Autodesk Fusion 360 part; units mm, degrees
sketch "スケッチ2" plane through (0, 0, 0) normal (0, 0, 1) x (1, 0, 0)
  line L0 (27.5, 37.5) -> (27.5, -37.5)
  line L1 (-27.5, -37.5) -> (-27.5, 37.5)
  arc A0 (27.5, 37.5) -> (-27.5, 37.5) centre (0, 37.5) ccw
  arc A1 (-27.5, -37.5) -> (27.5, -37.5) centre (0, -37.5) ccw
  dimension "d2" = 27.5
  dimension "d3" = 75
  dimension "d4" = 37.5
extrude "押し出し1" add sketch "スケッチ2" along normal blind 50
sketch "スケッチ3" plane through (0, 0, 50) normal (0, 0, 1) x (-1, 0, 0)
  arc A0 (-27.5, -37.5) -> (27.5, -37.5) centre (0, -37.5) ccw
  line L0 (27.5, -37.5) -> (27.5, 37.5)
  arc A1 (27.5, 37.5) -> (-27.5, 37.5) centre (0, 37.5) ccw
  line L1 (-27.5, 37.5) -> (-27.5, -37.5)
  line L2 (20, -29) -> (20, 20)
  arc A2 (20, 20) -> (-20, 20) centre (0, 20) ccw
  line L3 (-20, 20) -> (-20, -29)
  line L4 (-20, -29) -> (-12, -37)
  line L5 (-12, -37) -> (12, -37)
  line L6 (12, -37) -> (20, -29)
  dimension "d7" = 20
  dimension "d8" = 57
  dimension "d9" = 24
  dimension "d45" = 20
extrude "押し出し2" cut sketch "スケッチ3" against normal blind 20 contours L2 A2 L3 L4 L5 L6
sketch "スケッチ4" plane through (0, 0, 30) normal (0, 0, 1) x (-1, 0, 0)
  line L0 (12, -37) -> (20, -29)
  line L1 (20, -29) -> (20, 20)
  arc A0 (20, 20) -> (-20, 20) centre (0, 20) ccw
  line L2 (-20, 20) -> (-20, -29)
  line L3 (-20, -29) -> (-12, -37)
  line L4 (-12, -37) -> (12, -37)
  line L5 (10, -27) -> (-10, -27)
  line L6 (-10, -27) -> (-10, -7)
  line L7 (-10, -7) -> (10, -7)
  line L8 (10, -7) -> (10, -27)
  dimension "d14" = 10
  dimension "d48" = 10
  dimension "d49" = 10
extrude "押し出し3" cut sketch "スケッチ4" against normal blind 19 contours L5 L6 L7 L8
sketch "スケッチ5" plane through (0, 0, 0) normal (0, 1, 0) x (1, 0, 0)
  arc A0 (12, -9) -> (-12, -9) centre (0, -12.5) ccw
  line L0 (35, -41.8786) -> (35, 32.3347)
  line L1 (35, 32.3347) -> (-35, 32.3347)
  line L2 (-35, 32.3347) -> (-35, -41.8786)
  line L3 (75, -350) -> (-75, -350)
  line L4 (-27.5, 0) -> (27.5, 0)
  arc A1 (35, -41.8786) -> (12, -9) centre (0, -41.8786) ccw
  arc A2 (-12, -9) -> (-35, -41.8786) centre (0, -41.8786) ccw
  dimension "d18" = 12.5
  dimension "d19" = 350
  dimension "d23" = 70
  dimension "d24" = 35
revolve "回転1" cut sketch "スケッチ5" angle 360 about axis through (75, 0, 350) along (-1, 0, 0)
sketch "スケッチ9" plane through (10, 0, 0) normal (-1, 0, 0) x (0, -1, 0)
  line L0 (-7, 30) -> (-27, 30)
  line L1 (-27, 30) -> (-27, 11)
  line L2 (-27, 11) -> (-7, 11)
  line L3 (-7, 11) -> (-7, 30)
  circle A0 centre (-17, 21) radius 3.25
  dimension "d31" = 6.5
  dimension "d32" = 9
  dimension "d33" = 10
extrude "押し出し6" cut sketch "スケッチ9" along normal through all and the other way through all contours A0
sketch "スケッチ14" plane through (0, 0, 0) normal (1, 0, 0) x (0, 1, 0)
  circle A0 centre (17, 21) radius 8.544
  point P0 (17, 21)
  dimension "d40" = 17.088
extrude "押し出し8" cut sketch "スケッチ14" along normal blind 20 from surface at 20
mirror "ミラー1" about plane through (0, 0, 0) normal (1, 0, 0) of "押し出し8"
sketch "スケッチ15" plane through (0, 0, 50) normal (0, 0, 1) x (-1, 0, 0)
  line L0 (20, 20) -> (20, -29)
  line L1 (20, -29) -> (12, -37)
  line L2 (12, -37) -> (-12, -37)
  line L3 (-12, -37) -> (-20, -29)
  line L4 (-20, -29) -> (-20, 20)
  arc A0 (20, 20) -> (-20, 20) centre (0, 20) ccw
  arc A1 (-27.5, -37.5) -> (27.5, -37.5) centre (0, -37.5) ccw
  line L5 (27.5, -37.5) -> (27.5, 37.5)
  arc A2 (27.5, 37.5) -> (-27.5, 37.5) centre (0, 37.5) ccw
  line L6 (-27.5, 37.5) -> (-27.5, -37.5)
  line L7 (42.7311, -72.162) -> (-49.8708, -72.162)
  line L8 (-49.8708, -72.162) -> (-49.8708, 74.8211)
  line L9 (-49.8708, 74.8211) -> (42.7311, 74.8211)
  line L10 (42.7311, 74.8211) -> (42.7311, -72.162)
extrude "押し出し9" cut sketch "スケッチ15" against normal blind 15 contours A1 L5 A2 L6
CAD build for the part. Positions are in the model's coordinates, mm. A direction names the side the tool comes from. Coordinates: 2 decimals unless noted, no trailing zeros. Write each loop counter-clockwise with the first axis right and the second up, starting at its lowest first coordinate (ties: lowest second). Pieces come first, ordered by that corner, then holes.
(1) Flat gauge pins, fed straight in: pin 1 (1.5 mm diameter, centred on y = -16.5, z = 12, fed in from -X); pin 2 (8 mm diameter, centred on y = 15, z = 18, fed in from +X); pin 3 (22 mm diameter, centred on x = 2.5, y = 18.5, fed in from +Z). Where does each tip first touch, or does it go through?
(2) Cut at C-C, the plane y = 17. Count the separate pieces of the cut face and the enclosed holes in it, and give its area (3 significant figures).
(3) Cut at A-A, the plane x = 0. List the corners of the cut face in (y, z).
(4) Cut at B-B, the plane z = 25.5. List the corners of the cut face in (x, y), and give its area (3 significant figures).
(5) 3-axis set-ups, long thin cutter, end or side, ignore diameter. For faces 4 (the face through (20, 15, 18)), 5 (the face through (-23.697, 16.871, 29.543)), 6 (the face through (-20, 5, 33)): which of +Z, -Z, +X, -X, +Y, -Y reach the whole face in a straight line?
(6) Two-plate mould, pull along X, no slides. Class faces 1 (the face through (-14.93, 20.247, 20.857)), 2 (the face through (0, 7, 21)), 3 (the face through (27.5, 1, 28)): +X half, -X half, draft (parallel to the pull), parting line (faces both ways), or undercut.
(7) Drill centre lines: probe 1 along X at (y, z) = (22.5, 20); probe 2 along Y at (x, z) = (1, 18); probe 3 along Z at (x, y) = (-24.5, 17). Where is each one in solid material? Low to high.
Geometry says:
1. pin 1: stops at x = -18.79
1. pin 2: stops at x = 20
1. pin 3: stops at z = 30
2. separate pieces: 3
2. enclosed holes: 0
2. area: 524 mm2
3. outline: (-65, 6.09) arc R350 ccw to (65, 6.09) - (65, 35) - (37, 35) - (37, 30) - (27, 30) - (27, 11) - (7, 11) - (7, 30) - (-40, 30) - (-40, 35) - (-65, 35) - close
4. outline: (-27.5, -37.5) arc R27.5 ccw to (27.5, -37.5) - (27.5, 9.74) - (20, 9.74) - (20, 24.26) - (27.5, 24.26) - (27.5, 37.5) arc R27.5 ccw to (-27.5, 37.5) - (-27.5, 24.26) - (-20, 24.26) - (-20, 9.74) - (-27.5, 9.74) - close; hole (-10, 7) - (10, 7) - (10, 27) - (-10, 27) - close
4. area: 5,880 mm2
5. face 4: +X
5. face 5: -X
5. face 6: +Z
6. face 1: draft
6. face 2: undercut
6. face 3: +X half
7. probe 1: x = -20 to -10, 10 to 20
7. probe 2: y = -64.98 to 7, 27 to 64.98
7. probe 3: z = 29.54 to 35
